Study the drawing (mm; zero at the part's minimum x, y, z) and answer. Coordinates: 2 decimals unless noted, no trailing zeros. Loops run counter-clockwise (first coordinate to the right, second up) from the corner with the lowest first, then second, coordinate; pieces in that order, holes last. Notation, with made-up numbers: (86, 54) - (105, 54) arc R20 ccw to (105, 84) - close; hole circle Ø10 at (-31.5, -24). An arc over 180 degrees is marked (long way). Use one line per item in the form item = value. Start each with the question number.
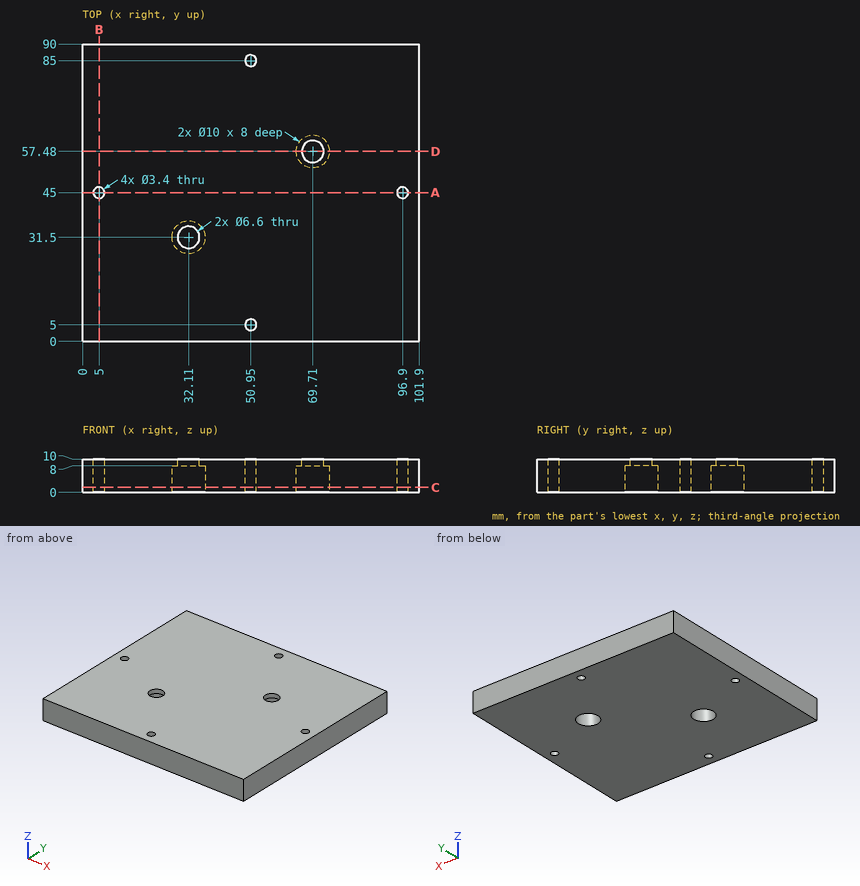
(1) A cutting plane is placed at D-D (y = 57.48). Determine the outline of the cut face in (x, z), then the cut area to 3 significant figures.
(2) A cutting plane is placed at C-C (z = 1.5). Determine the outline of the cut face in (x, y), then the cut area to 3 significant figures.
(3) This flat-tipped pin is pushed along its axis until it touches: pin 1 Ø8.5 at (x, y) = (32.11, 31.5) entering from -Z. Where does it stop, or does it pass through?
(4) Find the intervals of material crossed by probe 1 along Y at (x, z) = (50.95, 2.75); probe 2 along Y at (x, z) = (69.71, 8.75); probe 3 along X at (y, z) = (85, 5.25), in increasing order. Write a range as from..to.
(5) A cutting plane is placed at B-B (x = 5). Determine the outline of the cut face in (y, z).
(6) A cutting plane is placed at A-A (y = 45). Determine the outline of the cut face in (x, z), then the cut area to 3 significant figures.
Evaluation:
q1.outline = (0, 0) - (64.71, 0) - (64.71, 8) - (66.41, 8) - (66.41, 10) - (0, 10) - close; (73.01, 8) - (74.71, 8) - (74.71, 0) - (101.9, 0) - (101.9, 10) - (73.01, 10) - close
q1.area = 926 mm^2
q2.outline = (0, 0) - (101.9, 0) - (101.9, 90) - (0, 90) - close; hole circle Ø3.4 at (5, 45); hole circle Ø10 at (32.11, 31.5); hole circle Ø3.4 at (50.95, 5); hole circle Ø3.4 at (50.95, 85); hole circle Ø10 at (69.71, 57.48); hole circle Ø3.4 at (96.9, 45)
q2.area = 8,980 mm^2
q3.pin_1 = 8
q4.probe_1 = 0..3.3, 6.7..83.3, 86.7..90
q4.probe_2 = 0..54.18, 60.78..90
q4.probe_3 = 0..49.25, 52.65..101.9
q5.outline = (0, 0) - (43.3, 0) - (43.3, 10) - (0, 10) - close; (46.7, 0) - (90, 0) - (90, 10) - (46.7, 10) - close
q6.outline = (0, 0) - (3.3, 0) - (3.3, 10) - (0, 10) - close; (6.7, 0) - (95.2, 0) - (95.2, 10) - (6.7, 10) - close; (98.6, 0) - (101.9, 0) - (101.9, 10) - (98.6, 10) - close
q6.area = 951 mm^2
